from build123d import *

# Parameters (mm, degrees)
BOSS_EXTRUDE1_DEPTH  = 480
M4_CLEARANCE_HOLE1_D = 4.5
M4_CLEARANCE_HOLE2_D = 4.5


with BuildPart() as part:
    # Sketch1 → Boss-Extrude1 (new body)
    with BuildSketch(Plane.XY):
        Polygon((-65, 0), (65, 0), (65, 10.5), (50, 10.5), (50, 12), (-50, 12), (-50, 10.5), (-65, 10.5), align=None)
    extrude(amount=BOSS_EXTRUDE1_DEPTH)

    # M4 Clearance Hole1 (through all)
    with Locations(Plane(origin=(14.850423209, 10.5, 240), x_dir=(1, 0, 0), z_dir=(0, 1, 0))):
        with Locations((-72.350423209, -135), (-72.350423209, 225), (-72.350423209, -75), (-72.350423209, -15), (-72.350423209, 45), (-72.350423209, 105), (-72.350423209, 165)):
            Hole(M4_CLEARANCE_HOLE1_D / 2)

    # M4 Clearance Hole2 (through all)
    with Locations(Plane(origin=(14.850423209, 10.5, 240), x_dir=(1, 0, 0), z_dir=(0, 1, 0))):
        with Locations((42.649576791, -135), (42.649576791, 225), (42.649576791, -75), (42.649576791, -15), (42.649576791, 45), (42.649576791, 105), (42.649576791, 165)):
            Hole(M4_CLEARANCE_HOLE2_D / 2)


solid = part.part
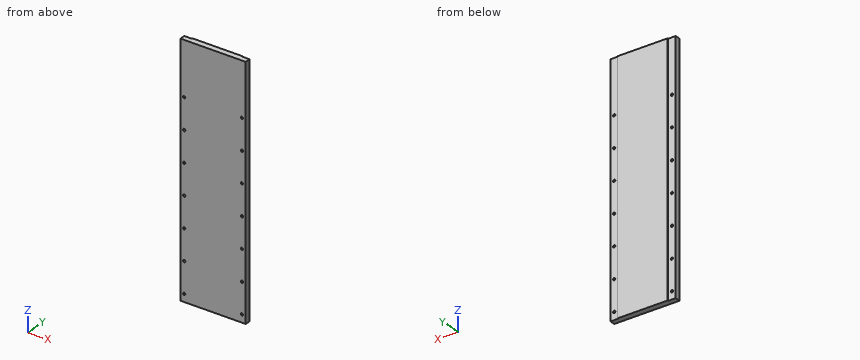
Model file for the job. Use its own axes, mm. Give positions to 0.01 mm unless a question says otherwise; leave off trailing zeros. Write each loop counter-clockwise with the first axis right and the second up, starting at its lowest first coordinate (ties: lowest second). Pieces come first, ordered by that corner, then holes. Notation, with made-up numbers: (45, 50) - (96, 50) arc R21 cw to (96, 71) - close; hole circle Ø7 at (53, -5). An arc over 180 degrees is marked (long way). Answer as CSV lines item,"result".
1. Band-saw the part on A-A (z = 210). Write the cut outline in (x, y), and give its area (4 significant figures).
Responses:
outline,"(-65, 0) - (65, 0) - (65, 10.5) - (50, 10.5) - (50, 12) - (-50, 12) - (-50, 10.5) - (-65, 10.5) - close"
area,"1,515 mm2"
2. Pin check, flat tips, straight feed: pin 1 (3.5 mm diameter, centred on x = 57.5, z = 255, fed in from +Y); pin 2 (7 mm diameter, centred on x = 57.5, z = 315, fed in from +Y). Stop position of each tip, or through.
Responses:
pin 1,"passes through"
pin 2,"stops at y = 10.5"
3. Drill centre lines: L1, parallel to X at y = 7, z = 195; L2, parallel to X at y = 11.5, z = 161; L3, parallel to Y at x = 59, z = 419. Where is each one in solid material? Low to high. Write a range as [from, to].
Responses:
L1,"x = [-65, -59.75], [-55.25, 55.25], [59.75, 65]"
L2,"x = [-50, 50]"
L3,"y = [0, 10.5]"
